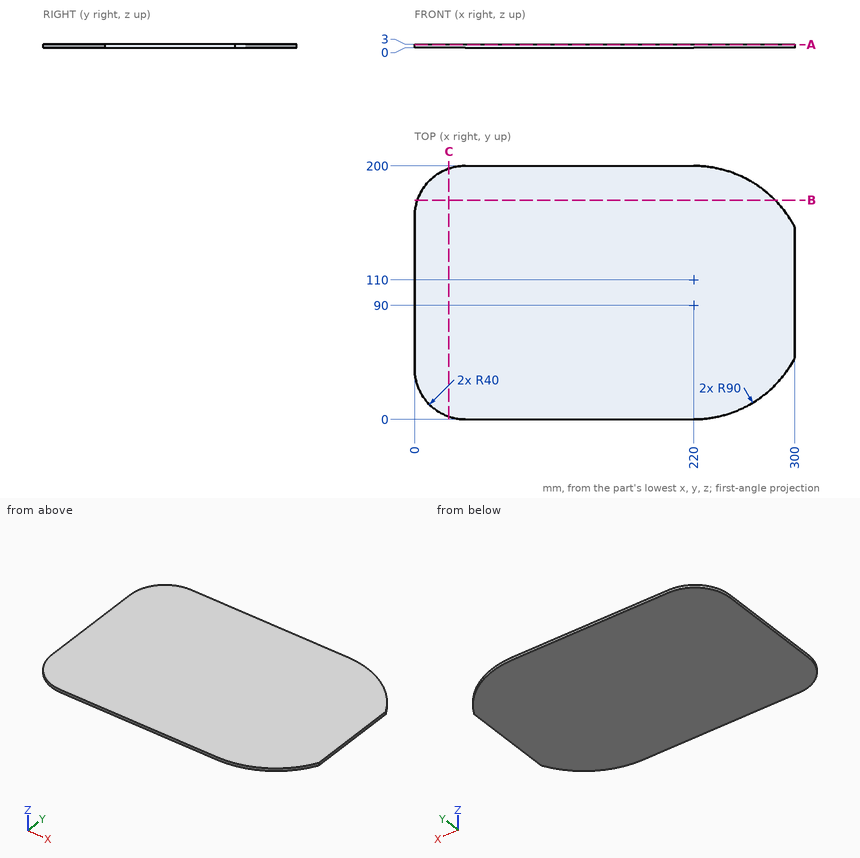
Could you check a few things on this drawing? It's one solid part, dimensions in mm from its lowest x, y, z. Coordinates: 2 decimals unless noted, no trailing zeros. Write each loop counter-clockwise with the first axis right and the second up, starting at its lowest first coordinate (ties: lowest second). Pieces come first, ordered by that corner, then holes. Notation, with made-up numbers: (-36, 80.5) - (-32, 80.5) arc R20 cw to (-32, 98.5) - close; hole circle Ø2 at (25.5, 13.5). An arc over 180 degrees is marked (long way). Put each result on its own line as item: value. Start each with the question number.
Q1. I want a section at B-B on y = 173. Write out the boundary of the cut face in (x, z), plus the area to 3 significant figures.
Q2. I want a section at C-C on x = 27. Write out the boundary of the cut face in (y, z).
Q3. I want a section at A-A on z = 2.55. Write out the boundary of the cut face in (x, y).
Q4. Please list where these lines run through material, in increasing order: L1, parallel to X at y = 14.5, z = 2.8; L2, parallel to X at y = 186.5, z = 1.05; L3, parallel to Y at x = 236, z = 2.05.
Checks:
1. outline: (2.17, 0) - (284.27, 0) - (284.27, 3) - (2.17, 3) - close
1. area: 846 mm²
2. outline: (2.17, 0) - (197.83, 0) - (197.83, 3) - (2.17, 3) - close
3. outline: (0, 40) arc R40 ccw to (40, 0) - (220, 0) arc R90 ccw to (300, 48.77) - (300, 151.23) arc R90 ccw to (220, 200) - (40, 200) arc R40 ccw to (0, 160) - close
4. L1: 9.18 to 268.99
4. L2: 10.04 to 267.41
4. L3: 1.43 to 198.57
